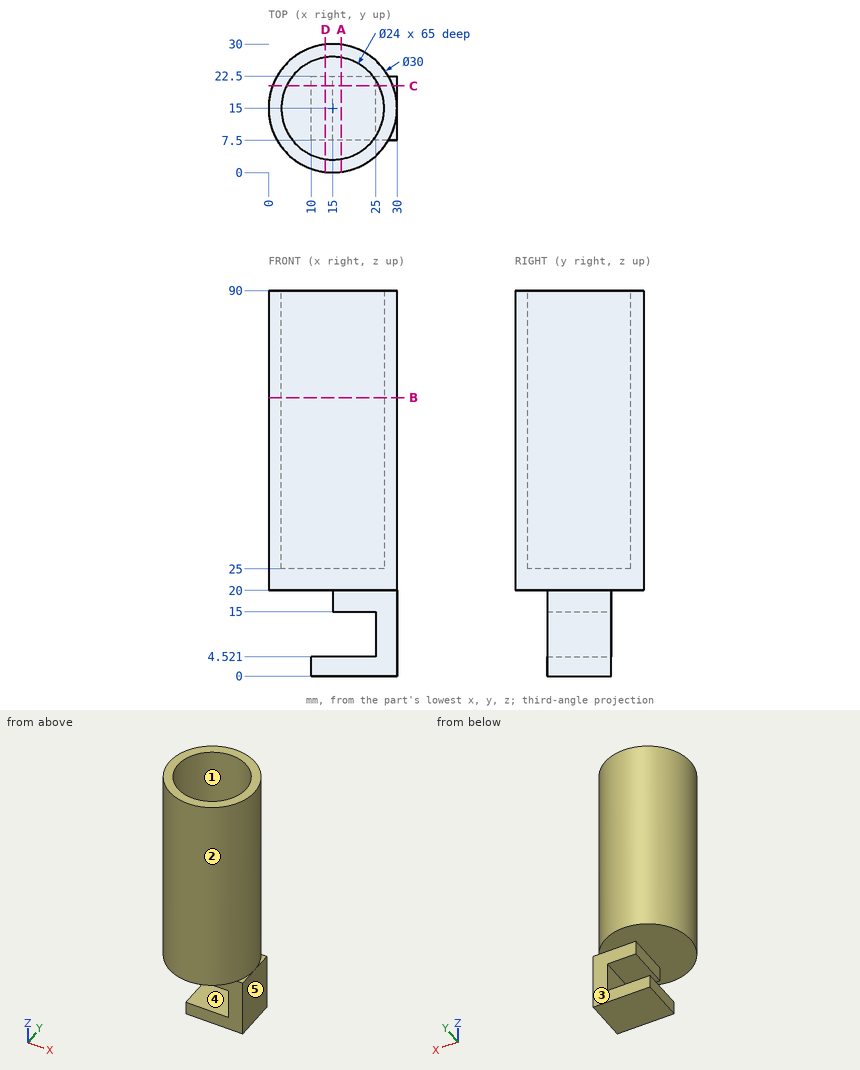
Input: dimensioned drawing with shaded views. Units: mm. Origin: part minimum x, y, z. A direction names the side the tool comes from. Coordinates: 2 decimals unless noted, no trailing zeros. Loops run counter-clockwise (first coordinate to the right, second up) from the corner with the lowest first, then second, coordinate; pieces in that order, holes last. Notation, with made-up numbers: M 28,-3.5 L 34,-3.5 A24 cw 34,11.5 Z; hole C -27.75,24.5 d10. An arc over 180 degrees is marked long. Put each result on its own line as item: value.
(1) Cut plane C-C on y = 20.25. Return the cut outline in (x, z).
Answer sheet:
outline: M 0.95,20 L 15,20 L 15,15 L 25,15 L 25,4.52 L 10,4.52 L 10,0 L 30,0 L 30,20 L 29.05,20 L 29.05,90 L 25.79,90 L 25.79,25 L 4.21,25 L 4.21,90 L 0.95,90 Z
(2) First-contact query: pin 1 (8 mm diameter, centred on x = 17.5, y = 21, fed in from +Z); pin 2 (16 mm diameter, centred on x = 19, z = 6, fed in from -Y); pin 3 (4 mm diameter, centred on y = 17.5, z = 18.5, fed in from -X). Flat tips, straight axial feed; report the tip coordinate or a pass-through.
Answer sheet:
pin 1: stops at z = 25
pin 2: stops at y = 7.5
pin 3: stops at x = 0.05
(3) Draft query along X for the marked faces 1, 2 and 3. Return one class per face: pulls with the +X half, pulls with the -X half, needs draft (parallel to the pull), parting line crosses it, or undercut.
Answer sheet:
face 1: undercut
face 2: parting line crosses it
face 3: needs draft
(4) Material intervals for probe 1 along Y at (x, z) = (15, 73); probe 2 along X at (y, z) = (5.25, 79) (1 decimal); probe 3 along Z at (x, y) = (17.5, 28.75), sorted ascending.
Answer sheet:
probe 1: y = 0 to 3, 27 to 30
probe 2: x = 3.6 to 8, 22 to 26.4
probe 3: z = 20 to 90
(5) Access query for the marked faces 4 and 5. Directions: +Z, -Z, +X, -X, +Y, -Y. A direction counts if a zero-diameter tool reaches every point of the face in a straight line with its end or side. Return the directions, or none.
Answer sheet:
face 4: -X, +Y, -Y
face 5: +Z, -Z, +X, +Y, -Y
(6) Cut plane B-B on z = 65. Return the cut outline in (x, y).
Answer sheet:
outline: C 15,15 d30; hole C 15,15 d24
(7) Cut plane A-A on x = 17. Return the cut outline in (y, z).
Answer sheet:
outline: M 0.13,20 L 7.5,20 L 7.5,15 L 22.5,15 L 22.5,20 L 29.87,20 L 29.87,90 L 26.83,90 L 26.83,25 L 3.17,25 L 3.17,90 L 0.13,90 Z; M 7.5,0 L 22.5,0 L 22.5,4.52 L 7.5,4.52 Z
(8) Cut plane D-D on x = 13.25. Return the cut outline in (y, z), then the cut area to 3 significant figures.
Answer sheet:
outline: M 0.1,20 L 29.9,20 L 29.9,90 L 26.87,90 L 26.87,25 L 3.13,25 L 3.13,90 L 0.1,90 Z; M 7.5,0 L 22.5,0 L 22.5,4.52 L 7.5,4.52 Z
area: 610 mm^2
